Source: three-view drawing plus pictorial views. Frame: mm from the lowest corner of the part. A direction names the side the tool comes from. Round coordinates to 2 decimals unless told otherwise and drop trailing zeros. Write each loop counter-clockwise with the first axis right and the second up, starting at its lowest first coordinate (ties: lowest second). Pieces come first, ordered by that corner, then holes. Notation, with made-up numbers: (-5.75, 68) -> (40.25, 68) arc R32 ccw to (40.25, 99) -> close; hole circle Ø10 at (35, 8). An arc over 180 degrees is marked (long way). Put each result on its own line as item: value.
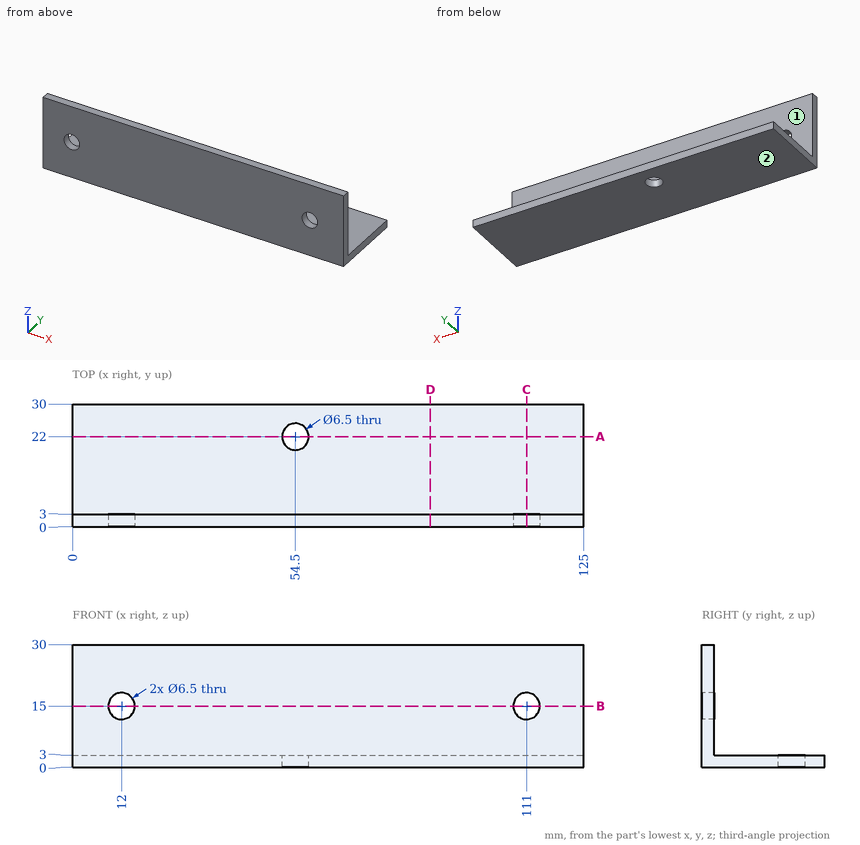
Q1. Cut plane A-A on y = 22. Output: boundary loops of the cut face in (x, z).
Ans:
outline: (0, 0) -> (51.25, 0) -> (51.25, 3) -> (0, 3) -> close; (57.75, 0) -> (125, 0) -> (125, 3) -> (57.75, 3) -> close
Q2. Cut plane B-B on z = 15. Output: boundary loops of the cut face in (x, y), and give its area (3 significant figures).
Ans:
outline: (0, 0) -> (8.75, 0) -> (8.75, 3) -> (0, 3) -> close; (15.25, 0) -> (107.75, 0) -> (107.75, 3) -> (15.25, 3) -> close; (114.25, 0) -> (125, 0) -> (125, 3) -> (114.25, 3) -> close
area: 336 mm^2
Q3. Cut plane D-D on x = 87.5. Output: boundary loops of the cut face in (y, z).
Ans:
outline: (0, 0) -> (30, 0) -> (30, 3) -> (3, 3) -> (3, 30) -> (0, 30) -> close
Q4. Cut plane C-C on x = 111. Output: boundary loops of the cut face in (y, z).
Ans:
outline: (0, 0) -> (30, 0) -> (30, 3) -> (3, 3) -> (3, 11.75) -> (0, 11.75) -> close; (0, 18.25) -> (3, 18.25) -> (3, 30) -> (0, 30) -> close
Q5. Material intervals for line 1 (X direction, y = 0.85, z = 15); line 2 (Z direction, x = 12, y = 1.6); line 3 (Z direction, x = 27, y = 25.5), sorted ascending. Write a range as [from, to].
Ans:
line 1: x = [0, 8.75], [15.25, 107.75], [114.25, 125]
line 2: z = [0, 11.75], [18.25, 30]
line 3: z = [0, 3]
Q6. Reachability of the marked faces 1 and 2 from +Z, -Z, +X, -X, +Y, -Y: full face, straight path, thin tool, end or side. Return the list, or none.
Ans:
face 1: +Z, +X, -X, +Y
face 2: -Z, +X, -X, +Y, -Y
Q7. Pin query (flat end, axial travel): pin 1 (5 mm diameter, centred on x = 76.5, z = 21, fed in from +Y); pin 2 (10 mm diameter, centred on x = 58, y = 4.5, fed in from +Z); pin 3 (6 mm diameter, centred on x = 111, z = 15, fed in from +Y); pin 4 (6 mm diameter, centred on x = 36.5, y = 22, fed in from +Z). Return the tip coordinate at first contact, or that it passes through.
Ans:
pin 1: stops at y = 3
pin 2: stops at z = 30
pin 3: passes through
pin 4: stops at z = 3
